Part model, mm, in its own coordinate system. A direction names the side the tool comes from. Round coordinates to 2 decimals unless told otherwise and drop trailing zeros. Write each loop counter-clockwise with the first axis right and the second up, starting at its lowest first coordinate (ties: lowest second). Pieces come first, ordered by that corner, then holes. Notation, with made-up numbers: (6, 66) -> (43, 66) arc R24 cw to (43, 80) -> close; hole circle Ø11 at (8.25, -9). An arc over 180 degrees is marked (long way). Use CSV: the item, a comma, the result in double quotes. Start each with the question number.
(1) Saw through at B-B (x = -54.5). Give the cut face in (y, z), plus the area to 3 significant figures.
(2) Saw through at D-D (y = 29.5). Give the cut face in (x, z), plus the area to 3 significant figures.
(3) Which spindle directions (+Z, -Z, +X, -X, +Y, -Y) get a long thin tool onto all of the face, cutting with end or side? Do faces 1 (the cylindrical face through (-40.28, 0.49, 0.99)), 2 (the flat face through (11, 0, 0)). Say none if no direction does.
(4) Saw through at C-C (z = 1.4). Count the separate pieces of the cut face and the enclosed holes in it, plus the area to 3 significant figures.
(5) Two-plate mould, pull along Y, no slides. Class faces 3 (the cylindrical face through (-14.681, -8.987, 0.986)), 4 (the flat face through (11, 0, 2)): released by +Y, released by -Y, zero draft, split by the parting line, or undercut.
(6) Probe line 1 (Y direction, x = -27, z = 0.3); line 2 (Y direction, x = -54.5, z = 1.15); line 3 (X direction, y = -4, z = 0.7). List the from-to ranges inside material, lowest first. Write a range as [from, to].
(7) Saw through at A-A (x = 50.5). Give the cut face in (y, z), plus the area to 3 significant figures.
```python
from build123d import *

# Parameters (mm, degrees)
CROQUIS1_W              = 115
CROQUIS1_H              = 65
SALIENTE_EXTRUIR1_DEPTH = 2
SALIENTE_EXTRUIR2_DEPTH = 2
CROQUIS3_R              = 1.5
CORTAR_EXTRUIR1_DEPTH   = 2
CROQUIS4_R              = 1.35
CROQUIS4_R_2            = 14.35
CROQUIS4_R_3            = 9.15
CORTAR_EXTRUIR3_DEPTH   = 2
CROQUIS5_R              = 1.366917162
SALIENTE_EXTRUIR3_DEPTH = 2
MATRIZC1_COUNT          = 5


with BuildPart() as part:
    # Croquis1 → Saliente-Extruir1 (new body)
    with BuildSketch(Plane.XY):
        Rectangle(CROQUIS1_W, CROQUIS1_H)
    extrude(amount=SALIENTE_EXTRUIR1_DEPTH)

    # Croquis2 → Saliente-Extruir2 (add)
    with BuildSketch(Plane(origin=(0, 0, 0), x_dir=(-1, 0, 0), z_dir=(0, 0, -1))):
        Polygon((-57.5, 32.5), (-77.5, -32.5), (-57.5, -32.5), align=None)
    extrude(amount=-SALIENTE_EXTRUIR2_DEPTH)

    # Croquis3 → Cortar-Extruir1 (cut)
    with BuildSketch(Plane(origin=(0, 0, 0), x_dir=(-1, 0, 0), z_dir=(0, 0, -1))):
        with Locations((-50.5, 29.5)):
            Circle(CROQUIS3_R)
        with Locations((-70.5, -29.5)):
            Circle(CROQUIS3_R)
        with Locations((54.5, -29.5)):
            Circle(CROQUIS3_R)
        with Locations((54.5, 29.5)):
            Circle(CROQUIS3_R)
    extrude(amount=-CORTAR_EXTRUIR1_DEPTH, mode=Mode.SUBTRACT)

    # Croquis4 → Cortar-Extruir3 (cut)
    # profile 1 of 5: a face of its own
    with BuildSketch(Plane(origin=(0, 0, 0), x_dir=(-1, 0, 0), z_dir=(0, 0, -1))):
        with Locations((13.94030488, 11.910589373)):
            Circle(CROQUIS4_R)
    # profile 2 of 5: a face of its own
    with BuildSketch(Plane(origin=(0, 0, 0), x_dir=(-1, 0, 0), z_dir=(0, 0, -1))):
        with Locations((37.94030488, 11.910589373)):
            Circle(CROQUIS4_R)
    # profile 3 of 5: a face of its own
    with BuildSketch(Plane(origin=(0, 0, 0), x_dir=(-1, 0, 0), z_dir=(0, 0, -1))):
        with Locations((37.94030488, -12.089410627)):
            Circle(CROQUIS4_R)
    # profile 4 of 5: a face of its own
    with BuildSketch(Plane(origin=(0, 0, 0), x_dir=(-1, 0, 0), z_dir=(0, 0, -1))):
        with Locations((13.94030488, -12.089410627)):
            Circle(CROQUIS4_R)
    # profile 5 of 5: a face of its own
    with BuildSketch(Plane(origin=(0, 0, 0), x_dir=(-1, 0, 0), z_dir=(0, 0, -1))):
        with Locations((25.94030488, -0.089410627)):
            Circle(CROQUIS4_R_2)
        with Locations((25.94030488, -0.089410627)):
            Circle(CROQUIS4_R_3, mode=Mode.SUBTRACT)
    extrude(amount=-CORTAR_EXTRUIR3_DEPTH, mode=Mode.SUBTRACT)


with BuildPart() as cortar_extruir3_piece_1:
    # of the separate pieces the step leaves, piece 1, a body of its own (cortar_extruir3_pieces)
    add(part.part.solids().sort_by_distance((-57.5, -32.5, 0))[0])



with BuildPart() as cortar_extruir3_piece_2:
    # of the separate pieces the step leaves, piece 2, a body of its own (cortar_extruir3_pieces)
    add(part.part.solids().sort_by_distance((-35.09030488, -0.089410627, 2))[0])


with BuildPart() as cortar_extruir3_piece_1_1:
    add(cortar_extruir3_piece_1.part)

    add(cortar_extruir3_piece_2.part)  # Saliente-Extruir3 merges Cortar-Extruir3 piece 2
    # Croquis5 → Saliente-Extruir3 (add)
    with BuildSketch(Plane.XY.offset(2)):
        with Locations((-25.94030488, -0.089410627)):
            Circle(CROQUIS5_R)
        with BuildLine():
            Line((-38.61837968, -6.811681029), (-34.227775342, -3.967597491))
            ThreePointArc((-34.227775342, -3.967597491), (-33.817608325, -4.744578769), (-33.334811119, -5.478638539))
            Line((-33.334811119, -5.478638539), (-37.159332333, -9.036808182))
            ThreePointArc((-37.159332333, -9.036808182), (-37.9405412, -7.958135318), (-38.61837968, -6.811681029))
        make_face()
    saliente_extruir3 = extrude(amount=-SALIENTE_EXTRUIR3_DEPTH)

    # MatrizC1: Saliente-Extruir3 ×5 about axis
    matrizc1_axis = Axis((-25.94030488, -0.089410627, 0), (0, 0, 1))
    for i in range(1, MATRIZC1_COUNT):
        add(saliente_extruir3.rotate(matrizc1_axis, i * 360 / MATRIZC1_COUNT))


solid = cortar_extruir3_piece_1_1.part
```
Answers:
1,outline,"(-32.5, 0) -> (-31, 0) -> (-31, 2) -> (-32.5, 2) -> close; (-28, 0) -> (28, 0) -> (28, 2) -> (-28, 2) -> close; (31, 0) -> (32.5, 0) -> (32.5, 2) -> (31, 2) -> close"
1,area,"118 mm²"
2,outline,"(-57.5, 0) -> (-56, 0) -> (-56, 2) -> (-57.5, 2) -> close; (-53, 0) -> (49, 0) -> (49, 2) -> (-53, 2) -> close; (52, 0) -> (58.42, 0) -> (58.42, 2) -> (52, 2) -> close"
2,area,"220 mm²"
3,face 1,"+Z, -Z"
3,face 2,"-Z, +X, -X, +Y, -Y"
4,separate pieces,"1"
4,enclosed holes,"13"
4,area,"7,750 mm²"
5,face 3,"undercut"
5,face 4,"zero draft"
6,line 1,"y = [-32.5, -14.4], [-9.18, 9], [14.22, 32.5]"
6,line 2,"y = [-32.5, -31], [-28, 28], [31, 32.5]"
6,line 3,"x = [-57.5, -39.75], [-34.28, -17.67], [-12.13, 68.73]"
7,outline,"(-32.5, 0) -> (28, 0) -> (28, 2) -> (-32.5, 2) -> close; (31, 0) -> (32.5, 0) -> (32.5, 2) -> (31, 2) -> close"
7,area,"124 mm²"
